```python
from build123d import *

# Parameters (mm, degrees)
SKETCH1_R            = 5
BOSS_EXTRUDE1_DEPTH  = 10
M3_CLEARANCE_HOLE1_D = 3.4


with BuildPart() as part:
    # Sketch1 → Boss-Extrude1 (new body)
    with BuildSketch(Plane.XY):
        Polygon((0, 0), (20, 0), (20, 14), (6, 14), (6, 4), (0, 4), align=None)
        with Locations((13, 7)):
            Circle(SKETCH1_R, mode=Mode.SUBTRACT)
    extrude(amount=BOSS_EXTRUDE1_DEPTH)

    # M3 Clearance Hole1 (through all)
    with Locations(Plane(origin=(0, 4, 0), x_dir=(-1, 0, 0), z_dir=(0, 1, 0))):
        with Locations((-3, 5)):
            Hole(M3_CLEARANCE_HOLE1_D / 2)


solid = part.part
```
Could you check a few things on this model? Use its own coordinates, in mm. A direction names the side the tool comes from. Round coordinates to 2 decimals unless told otherwise and drop trailing zeros. Loops run counter-clockwise (first coordinate to the right, second up) from the corner with the lowest first, then second, coordinate; pieces in that order, holes last. Notation, with made-up numbers: (17.25, 9) - (41.25, 9) arc R25 ccw to (41.25, 31) - close; hole circle Ø4 at (83.5, 89.5). An arc over 180 degrees is marked (long way). Answer in a Markdown table with one row per item. Add a question column.
(1) If we section it at C-C (y = 7): Please give me the cut outline in (x, z).
(2) If we section it at B-B (x = 13): Please give me the cut outline in (y, z), plus the area to 3 significant figures.
(3) If we section it at A-A (z = 5): Please give me the cut outline in (x, y).
(4) I need wall thicknesses on line 1 along Y through (x, z) = (13, 8.25); line 2 along Z through (x, y) = (3, 1.2); line 3 along X through (y, z) = (7.5, 2.25). Which ranges of each line are inside material? Lowest first, please.
(5) If we section it at D-D (y = 1): Please give me the cut outline in (x, z).
(6) If we mould it in two halves opening along Z, with no side actions, what happens to faces 3 (the face through (3.8, 2, 3.5)), 4 (the face through (13, 14, 5)), 5 (the face through (7.6, 5.5, 0))? For each: pulls with the +Z half, pulls with the -Z half, needs draft (parallel to the pull), parting line crosses it, or undercut.
(7) I'm going to push flat-ended pins straight in: pin 1 (4 mm diameter, centred on y = 8, z = 8.5, fed in from -X); pin 2 (5 mm diameter, centred on x = 2.5, z = 4, fed in from +Y). Where does each tip first touch, or does it pass through?
(8) For faces 1 (the face through (5, 4, 5)), 2 (the face through (17.77, 8.5, 4.93)), which set-ups out of +Z, -Z, +X, -X, +Y, -Y let a thin tool reach every point of the face, with its end or its side?
Model answer:
| question | item | result |
|---|---|---|
| 1 | outline | (6, 0) - (8, 0) - (8, 10) - (6, 10) - close; (18, 0) - (20, 0) - (20, 10) - (18, 10) - close |
| 2 | outline | (0, 0) - (2, 0) - (2, 10) - (0, 10) - close; (12, 0) - (14, 0) - (14, 10) - (12, 10) - close |
| 2 | area | 40.0 mm² |
| 3 | outline | (0, 0) - (1.3, 0) - (1.3, 4) - (0, 4) - close; (4.7, 0) - (20, 0) - (20, 14) - (6, 14) - (6, 4) - (4.7, 4) - close; hole circle Ø10 at (13, 7) |
| 4 | line 1 | y = 0 to 2, 12 to 14 |
| 4 | line 2 | z = 0 to 3.3, 6.7 to 10 |
| 4 | line 3 | x = 6 to 8.03, 17.97 to 20 |
| 5 | outline | (0, 0) - (20, 0) - (20, 10) - (0, 10) - close; hole circle Ø3.4 at (3, 5) |
| 6 | face 3 | undercut |
| 6 | face 4 | needs draft |
| 6 | face 5 | pulls with the -Z half |
| 7 | pin 1 | stops at x = 6 |
| 7 | pin 2 | stops at y = 4 |
| 8 | face 1 | +Z, -Z, -X, +Y |
| 8 | face 2 | +Z, -Z |
